Model file for the job. Use its own axes, mm. A direction names the side the tool comes from. Round coordinates to 2 decimals unless told otherwise and drop trailing zeros. Loops run counter-clockwise (first coordinate to the right, second up) from the corner with the lowest first, then second, coordinate; pieces in that order, holes last. Notation, with made-up numbers: (-24.5, 72) - (34.5, 72) arc R16 ccw to (34.5, 94) - close; hole circle Ø1 at (32, 89). An arc over 180 degrees is marked (long way). Answer as a JSON object with one key per item and string values.
from build123d import *

# Parameters (mm, degrees)
F0_R     = 3.5
F1_DEPTH = 1


with BuildPart() as f1:
    # F0 (on Top) → F1 (new body)
    with BuildSketch(Plane.XY):
        Polygon((0, -15), (-30, 0), (-30, -15), (0, -30), align=None)
        Polygon((30, 0), (0, -15), (0, -30), (30, -15), align=None)
        with BuildLine():
            Line((38, 0), (30, 0))
            Line((30, 0), (30, -15))
            Line((30, -15), (38, -15))
            ThreePointArc((38, -15), (45.5, -7.5), (38, 0))
        make_face()
        with Locations((38, -7.5)):
            Circle(F0_R, mode=Mode.SUBTRACT)
        with BuildLine():
            Line((-30, -15), (-30, 0))
            Line((-30, 0), (-38, 0))
            ThreePointArc((-38, 0), (-45.5, -7.5), (-38, -15))
            Line((-38, -15), (-30, -15))
        make_face()
        with Locations((-38, -7.5)):
            Circle(F0_R, mode=Mode.SUBTRACT)
    extrude(amount=F1_DEPTH)


solid = f1.part
1) Tool access for faces 4 (the flat face through (14.8, -22.6, 0.5)), 5 (the flat face through (-14.8, -7.6, 0.5)): list every direction of +Z, -Z, +X, -X, +Y, -Y with a clear straight run to the whole face (end or side of a thin tool).
Values follow:
{"face 4": "+Z, -Z, +X, -Y", "face 5": "+Z, -Z, +Y"}
2) Slice it at A-A on y = -7.5. List the corners of the cut face in (x, z), then the cut area to 3 significant figures.
Values follow:
{"outline": "(-45.5, 0) - (-41.5, 0) - (-41.5, 1) - (-45.5, 1) - close; (-34.5, 0) - (-15, 0) - (-15, 1) - (-34.5, 1) - close; (15, 0) - (34.5, 0) - (34.5, 1) - (15, 1) - close; (41.5, 0) - (45.5, 0) - (45.5, 1) - (41.5, 1) - close", "area": "47.0 mm²"}
3) Two-plate mould, pull along Y, no slides. Class faces 1 (the cylindrical face through (35.2, -9.6, 0.5)), 2 (the cylindrical face through (45.5, -7.66, 0.49)), 3 (the flat face through (-1, -15, 1)): pulls with the +Y half, pulls with the -Y half, needs draft (parallel to the pull), parting line crosses it, or undercut.
Values follow:
{"face 1": "undercut", "face 2": "parting line crosses it", "face 3": "needs draft"}
4) Drop a flat-ended pin along its axis: P1, Ø11, axis at x = -38, y = -7.5, coming from the +Z side. Give the stop position or say it passes through.
Values follow:
{"P1": "z = 1"}
5) Slice it at B-B on y = -2.25. List the corners of the cut face in (x, z).
Values follow:
{"outline": "(-43.36, 0) - (-25.5, 0) - (-25.5, 1) - (-43.36, 1) - close; (25.5, 0) - (43.36, 0) - (43.36, 1) - (25.5, 1) - close"}
6) Probe probe 1 along X at (y, z) = (-9.25, 0.6); probe 2 along Y at (x, z) = (37, 0.3); probe 3 along X at (y, z) = (-5.75, 0.2). List the from-to ranges inside material, lowest first.
Values follow:
{"probe 1": "-45.29 to -41.03, -34.97 to -11.5, 11.5 to 34.97, 41.03 to 45.29", "probe 2": "-15 to -10.85, -4.15 to 0", "probe 3": "-45.29 to -41.03, -34.97 to -18.5, 18.5 to 34.97, 41.03 to 45.29"}
7) Slice it at C-C on x = -32. List the corners of the cut face in (y, z), then the cut area to 3 significant figures.
Values follow:
{"outline": "(-15, 0) - (0, 0) - (0, 1) - (-15, 1) - close", "area": "15.0 mm²"}
8) Slice it at D-D on y = -25. List the corners of the cut face in (x, z).
Values follow:
{"outline": "(-10, 0) - (10, 0) - (10, 1) - (-10, 1) - close"}
